Verification items for this drawing (mm, ordinates from the low corner). Give positions to 0.01 mm unless a question says otherwise; leave off trailing zeros. Write each loop counter-clockwise with the first axis right and the second up, starting at its lowest first coordinate (ties: lowest second). Pieces come first, ordered by that corner, then holes. Notation, with made-up numbers: (-37.75, 28.5) -> (-20.75, 28.5) arc R22 cw to (-20.75, 45.5) -> close; hole circle Ø5 at (13.5, 87). An arc over 180 degrees is marked (long way). One line per item, written item: value.
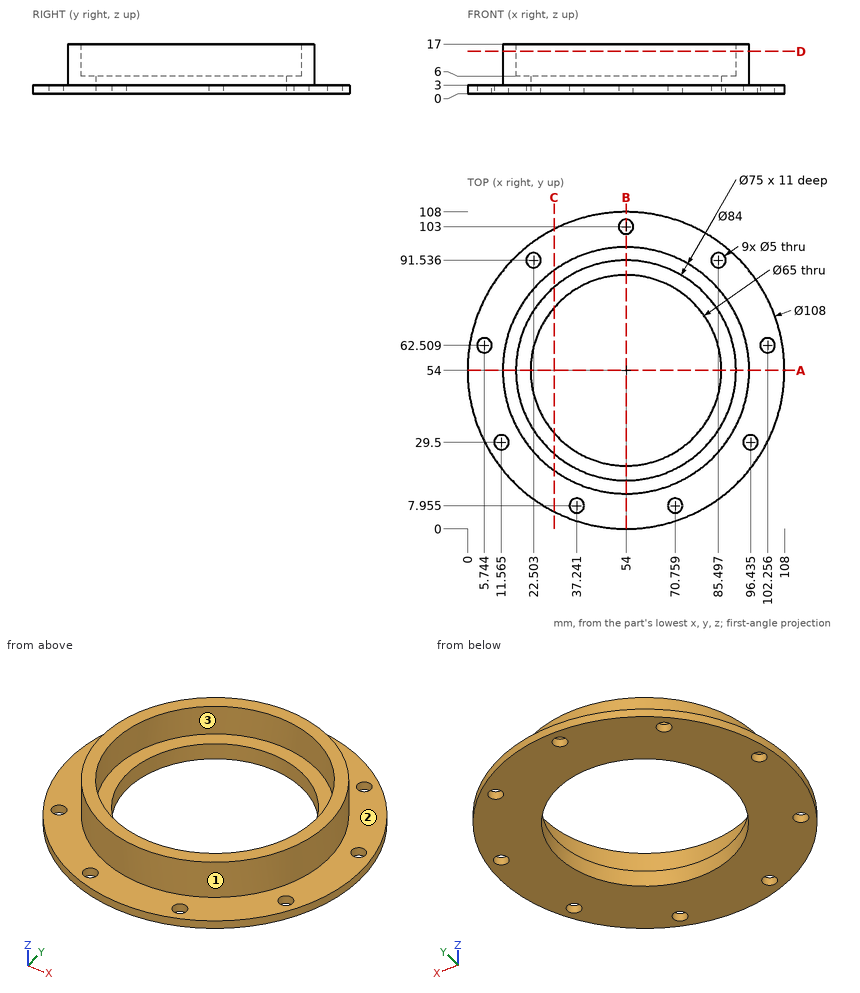
1) Scan lines: probe 1 along Z at (x, y) = (12, 38); probe 2 along X at (y, z) = (29, 11.5); probe 3 along X at (y, z) = (52, 11.75). Record each from-to range of solid material in increasing order.
Verdict:
probe 1: 0 to 3
probe 2: 20.25 to 26.05, 81.95 to 87.75
probe 3: 12.05 to 16.55, 91.45 to 95.95
2) Mould release check, pull along Y, two halves, no side actions. Record for the marked faces 1, 2 and 3: released by +Y, released by -Y, zero draft, split by the parting line, or undercut.
Verdict:
face 1: split by the parting line
face 2: zero draft
face 3: undercut
3) Sectioned sample at D-D on z = 14.5. Record the cut outline in (x, y), plus the area to 3 significant figures.
Verdict:
outline: circle Ø84 at (54, 54); hole circle Ø75 at (54, 54)
area: 1,120 mm^2
4) Sectioned sample at A-A on y = 54. Record the cut outline in (x, z), plus the area to 3 significant figures.
Verdict:
outline: (0, 0) -> (21.5, 0) -> (21.5, 6) -> (16.5, 6) -> (16.5, 17) -> (12, 17) -> (12, 3) -> (0, 3) -> close; (86.5, 0) -> (108, 0) -> (108, 3) -> (96, 3) -> (96, 17) -> (91.5, 17) -> (91.5, 6) -> (86.5, 6) -> close
area: 285 mm^2
5) Sectioned sample at C-C on x = 29.5. Record the cut outline in (y, z) (1 decimal).
Verdict:
outline: (5.9, 0) -> (32.6, 0) -> (32.6, 6) -> (25.6, 6) -> (25.6, 17) -> (19.9, 17) -> (19.9, 3) -> (5.9, 3) -> close; (75.4, 0) -> (102.1, 0) -> (102.1, 3) -> (88.1, 3) -> (88.1, 17) -> (82.4, 17) -> (82.4, 6) -> (75.4, 6) -> close
6) Depth check by flat-ended pin: pin 1 Ø4 at (x, z) = (16, 5.5) entering from -Y (1 decimal); pin 2 Ø6 at (x, y) = (37.24, 7.96) entering from -Z; pin 3 Ø10 at (x, z) = (59.5, 2) entering from -Y; pin 4 Ø6 at (x, z) = (63.5, 4) entering from +Y. Enter the tip coordinate at first touch or a pass-through.
Verdict:
pin 1: y = 32.4
pin 2: z = 0
pin 3: y = 0
pin 4: y = 107.59
7) Sectioned sample at B-B on x = 54. Record the cut outline in (y, z), plus the area to 3 significant figures.
Verdict:
outline: (0, 0) -> (21.5, 0) -> (21.5, 6) -> (16.5, 6) -> (16.5, 17) -> (12, 17) -> (12, 3) -> (0, 3) -> close; (86.5, 0) -> (100.5, 0) -> (100.5, 3) -> (96, 3) -> (96, 17) -> (91.5, 17) -> (91.5, 6) -> (86.5, 6) -> close; (105.5, 0) -> (108, 0) -> (108, 3) -> (105.5, 3) -> close
area: 270 mm^2
